Part model, mm, in its own coordinate system. A direction names the side the tool comes from. Coordinates: 2 decimals unless noted, no trailing zeros. Loops run counter-clockwise (first coordinate to the right, second up) from the corner with the lowest first, then second, coordinate; pieces in that order, holes last. Notation, with made-up numbers: M 4,40.25 L 12,40.25 A21 ccw 12,58.25 Z; hole C -18,-13 d5. An arc over 180 degrees is marked long. Answer as CSV lines item,"result". Start each with the question number.
from build123d import *

# Parameters (mm, degrees)
SKETCH1_R           = 19.05
BOSS_EXTRUDE1_DEPTH = 7.62
SKETCH2_R           = 9.398
BOSS_EXTRUDE2_DEPTH = 4.699
SKETCH7_R           = 2.921
CUT_EXTRUDE5_DEPTH  = 10.16
SKETCH12_R          = 1.5875
CUT_EXTRUDE6_DEPTH  = 3.159
CUT_EXTRUDE7_DEPTH  = 5.08
SKETCH14_R          = 1.27
CUT_EXTRUDE8_DEPTH  = 8.62


with BuildPart() as part:
    # Sketch1 → Boss-Extrude1 (new body)
    with BuildSketch(Plane(origin=(0, 0, 0), x_dir=(1, 0, 0), z_dir=(0, 1, 0))):
        Circle(SKETCH1_R)
    extrude(amount=BOSS_EXTRUDE1_DEPTH)

    # Sketch2 → Boss-Extrude2 (add)
    with BuildSketch(Plane(origin=(0, 7.62, 0), x_dir=(1, 0, 0), z_dir=(0, 1, 0))):
        Circle(SKETCH2_R)
    extrude(amount=BOSS_EXTRUDE2_DEPTH)

    # Sketch7 → Cut-Extrude5 (cut)
    with BuildSketch(Plane.XZ):
        with Locations((0, 5.08)):
            Circle(SKETCH7_R)
        with Locations((0, -5.08)):
            Circle(SKETCH7_R)
    extrude(amount=-CUT_EXTRUDE5_DEPTH, mode=Mode.SUBTRACT)

    # Sketch12 → Cut-Extrude6 (cut, through all)
    with BuildSketch(Plane.XZ.offset(-10.16)):
        with Locations((0, 5.08)):
            Circle(SKETCH12_R)
        with Locations((0, -5.08)):
            Circle(SKETCH12_R)
    extrude(amount=-CUT_EXTRUDE6_DEPTH, mode=Mode.SUBTRACT)

    # Sketch13 → Cut-Extrude7 (cut)
    with BuildSketch(Plane(origin=(0, 7.62, 0), x_dir=(1, 0, 0), z_dir=(0, 1, 0))):
        Polygon((2.346351494, 12.7), (1.173175747, 14.732), (-1.173175747, 14.732), (-2.346351494, 12.7), (-1.173175747, 10.668), (1.173175747, 10.668), align=None)
        Polygon((2.346351494, -12.7), (1.173175747, -10.668), (-1.173175747, -10.668), (-2.346351494, -12.7), (-1.173175747, -14.732), (1.173175747, -14.732), align=None)
        Polygon((15.046351494, 0), (13.873175747, 2.032), (11.526824253, 2.032), (10.353648506, 0), (11.526824253, -2.032), (13.873175747, -2.032), align=None)
        Polygon((-10.353648506, 0), (-11.526824253, 2.032), (-13.873175747, 2.032), (-15.046351494, 0), (-13.873175747, -2.032), (-11.526824253, -2.032), align=None)
    extrude(amount=-CUT_EXTRUDE7_DEPTH, mode=Mode.SUBTRACT)

    # Sketch14 → Cut-Extrude8 (cut, through all)
    with BuildSketch(Plane(origin=(0, 7.62, 0), x_dir=(1, 0, 0), z_dir=(0, 1, 0))):
        with Locations((0, 12.7)):
            Circle(SKETCH14_R)
        with Locations((12.7, 0)):
            Circle(SKETCH14_R)
        with Locations((0, -12.7)):
            Circle(SKETCH14_R)
        with Locations((-12.7, 0)):
            Circle(SKETCH14_R)
    extrude(amount=-CUT_EXTRUDE8_DEPTH, mode=Mode.SUBTRACT)


solid = part.part
Q1. Slice it at A-A, the plane y = 1. Write the cut outline in (x, z).
Q2. Wall check: L1, parallel to Z at x = 0, y = 0.6; L2, parallel to Z at x = 0, y = 7.75; L3, parallel to Y at x = -17, z = 5. Give the ranges that are in metal, low to high.
Q3. Tool access for faces 1 (the face through (-13.97, 1.29, -0.06)), 2 (the face through (14.47, 5.12, -1)), 3 (the face through (-2.153, 5.009, -3.106)): list every direction of +Z, -Z, +X, -X, +Y, -Y with a clear straight run to the whole face (end or side of a thin tool).
Q4. Slice it at B-B, the plane x = -12.7. Write the cut outline in (y, z), and give its area (3 significant figures).
Q5. Slice it at D-D, the plane x = 0. State how many separate pieces and enclosed holes the cut face has, and give its area (3 significant figures).
Q6. Two-plate mould, pull along Z, no slides. Class faces 4 (the face through (0, 12.319, 0)), 5 (the face through (-0.28, 1.29, 13.94)): +Z half, -Z half, draft (parallel to the pull), parting line (faces both ways), or undercut.
Q7. Slice it at C-C, the plane z = 5.08. Write the cut outline in (x, y), and give its area (3 significant figures).
Q8. Flat gauge pins, fed straight in: P1, Ø1.9, axis at x = 0, y = 4, coming from the +Z side; P2, Ø2, axis at x = 4.5, y = 2.5, coming from the +Z side; P3, Ø5, axis at x = 14, z = -2.5, coming from the +Y side; P4, Ø1.5, axis at x = 0, z = 12.7, coming from the +Y side. Where does each tip first touch, or does it go through?
Solved:
1,outline,"C 0,0 d38.1; hole C -12.7,0 d2.54; hole C 0,-5.08 d5.84; hole C 0,5.08 d5.84; hole C 0,-12.7 d2.54; hole C 0,12.7 d2.54; hole C 12.7,0 d2.54"
2,L1,"z = -19.05 to -13.97, -11.43 to -8, -2.16 to 2.16, 8 to 11.43, 13.97 to 19.05"
2,L2,"z = -9.4 to -8, -2.16 to 2.16, 8 to 9.4"
2,L3,"y = 0 to 7.62"
3,face 1,"+Y, -Y"
3,face 2,"+Y"
3,face 3,"-Y"
4,outline,"M 0,-14.2 L 7.62,-14.2 L 7.62,-2.03 L 2.54,-2.03 L 2.54,-1.27 L 0,-1.27 Z; M 0,1.27 L 2.54,1.27 L 2.54,2.03 L 7.62,2.03 L 7.62,14.2 L 0,14.2 Z"
4,area,"189 mm2"
5,separate pieces,"5"
5,enclosed holes,"0"
5,area,"192 mm2"
6,face 4,"draft"
6,face 5,"undercut"
7,outline,"M -18.36,0 L -2.92,0 L -2.92,10.16 L -1.59,10.16 L -1.59,12.32 L -7.91,12.32 L -7.91,7.62 L -18.36,7.62 Z; M 1.59,10.16 L 2.92,10.16 L 2.92,0 L 18.36,0 L 18.36,7.62 L 7.91,7.62 L 7.91,12.32 L 1.59,12.32 Z"
7,area,"288 mm2"
8,P1,"stops at z = 19.05"
8,P2,"stops at z = 18.73"
8,P3,"stops at y = 7.62"
8,P4,"passes through"
